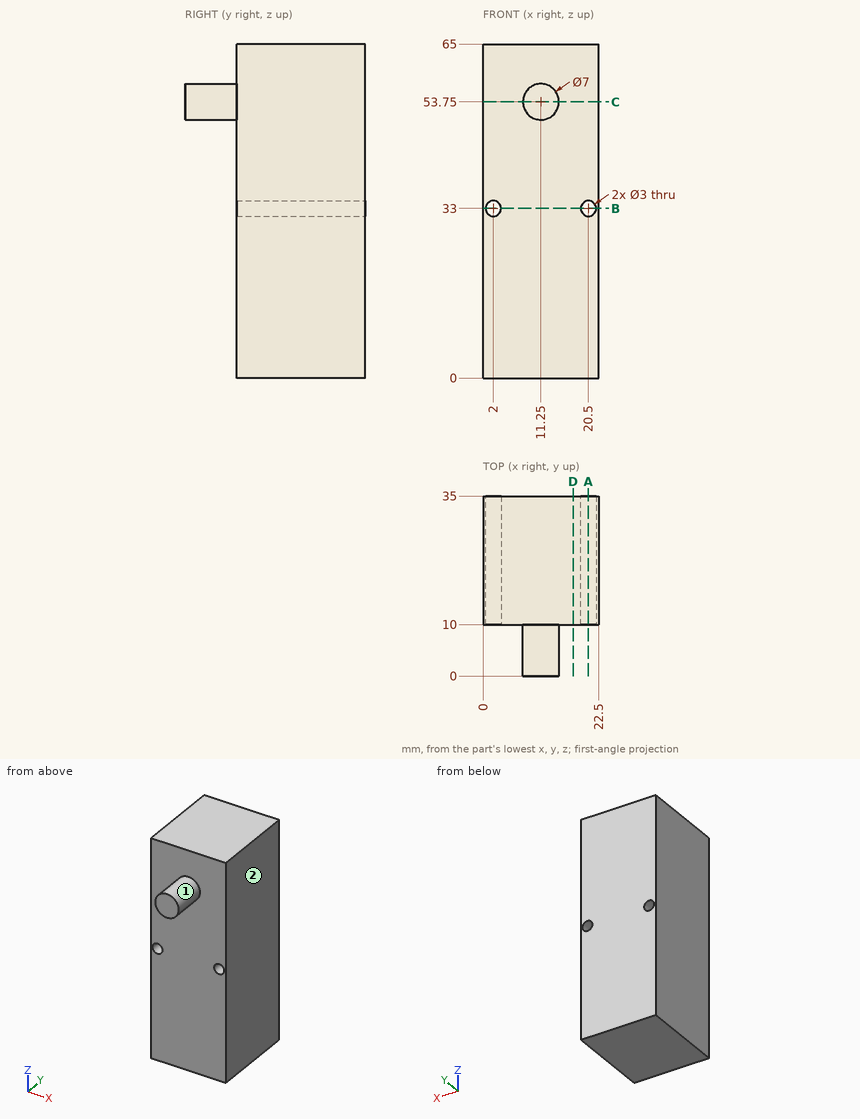
Check sheet for the drawn part. Datum: minimum x, y, z corner. Units: mm. A direction names the side the tool comes from. Round coordinates to 2 decimals unless told otherwise and drop trailing zeros. Write each loop counter-clockwise with the first axis right and the second up, starting at its lowest first coordinate (ties: lowest second). Pieces come first, ordered by that corner, then holes. Notation, with made-up numbers: (75.5, 21.5) -> (104.5, 21.5) arc R21 ccw to (104.5, 39.5) -> close; hole circle Ø4 at (75.5, 63). An arc over 180 degrees is marked (long way). Put each result on its own line as item: value.
(1) Sectioned sample at A-A (x = 20.5). Enter the section's corners in (y, z), plus the area to 3 significant figures.
Values found:
outline: (10, 0) -> (35, 0) -> (35, 31.5) -> (10, 31.5) -> close; (10, 34.5) -> (35, 34.5) -> (35, 65) -> (10, 65) -> close
area: 1,550 mm^2
(2) Material ranges on line 1 (Z direction, x = 2, y = 17.75); line 2 (Y direction, x = 11.5, z = 62.5), recorded low to high.
Values found:
line 1: z = 0 to 31.5, 34.5 to 65
line 2: y = 10 to 35
(3) Sectioned sample at C-C (z = 53.75). Enter the section's corners in (x, y).
Values found:
outline: (0, 10) -> (7.75, 10) -> (7.75, 0) -> (14.75, 0) -> (14.75, 10) -> (22.5, 10) -> (22.5, 35) -> (0, 35) -> close
(4) Sectioned sample at D-D (x = 17.5). Enter the section's corners in (y, z), plus the area to 4 significant figures.
Values found:
outline: (10, 0) -> (35, 0) -> (35, 65) -> (10, 65) -> close
area: 1,625 mm^2
(5) Go/stop test with flat-tipped pins: pin 1 Ø11 at (x, z) = (13, 37) entering from -Y; pin 2 Ø2 at (y, z) = (6, 52.5) entering from -X. Record where each tip stops, or that it passes through.
Values found:
pin 1: stops at y = 10
pin 2: stops at x = 7.76
(6) Tool access check on the marked faces 1 and 2. Record the directions out of +Z, -Z, +X, -X, +Y, -Y that give a thin tool (end or side, any length) a straight path to the whole face; none if there is none.
Values found:
face 1: -Y
face 2: +Z, -Z, +X, +Y, -Y
(7) Sectioned sample at B-B (z = 33). Enter the section's corners in (x, y).
Values found:
outline: (0, 10) -> (0.5, 10) -> (0.5, 35) -> (0, 35) -> close; (3.5, 10) -> (19, 10) -> (19, 35) -> (3.5, 35) -> close; (22, 10) -> (22.5, 10) -> (22.5, 35) -> (22, 35) -> close
